Here's the drawing with two shaded views (mm, measured from the low corner). I have some questions. Round coordinates to 2 decimals unless told otherwise and drop trailing zeros. Order: outer loops, then holes, each group sorted by start corner. A loop starts at its lowest first (then second) coordinate and runs counter-clockwise, first axis right, second up. Notation, with made-up numbers: (18.5, 70) -> (47.5, 70) arc R22 ccw to (47.5, 106) -> close; hole circle Ø4 at (62.5, -6.75). An arc over 180 degrees is marked (long way). One line per question, with ' | ' between items.
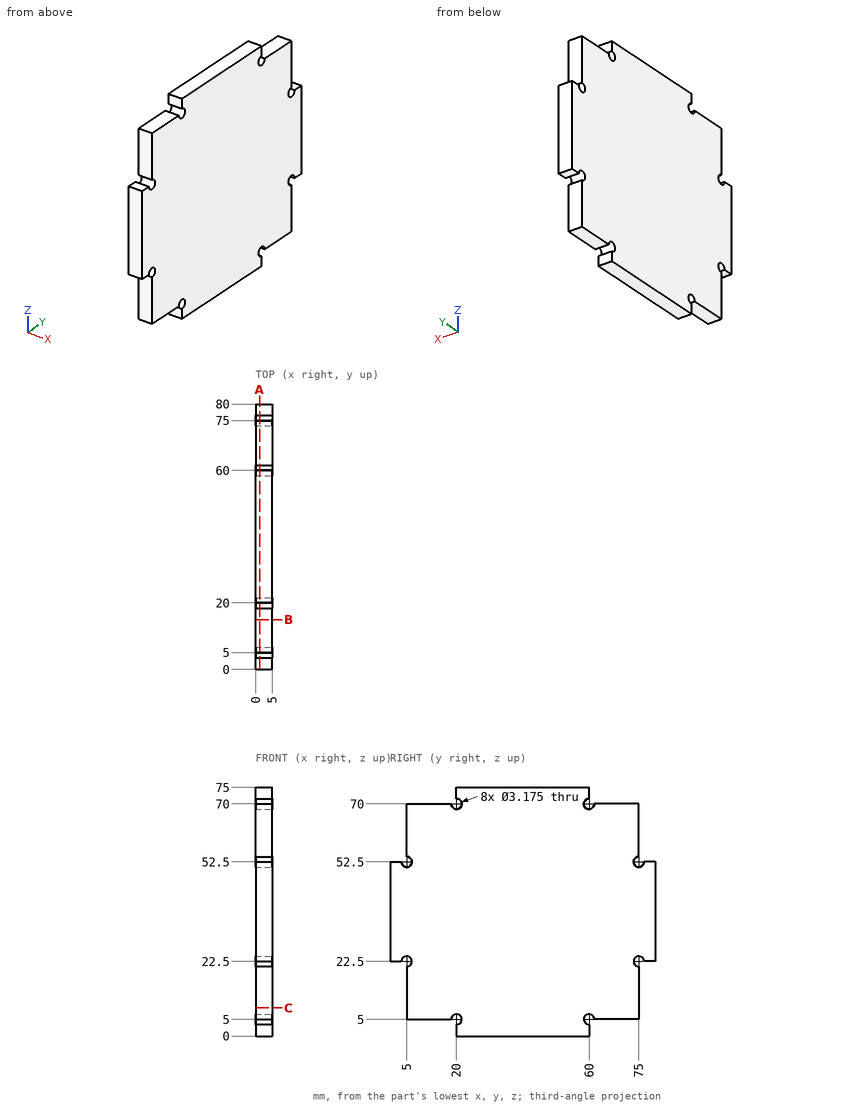
1. I need wall thicknesses on probe 1 along Z at (x, y) = (0.3, 17); probe 2 along Z at (x, y) = (4.65, 20.5); probe 3 along Y at (x, z) = (3.3, 62). Which ranges of each line are inside material? Lowest first, please.
From the geometry:
probe 1: z = 5 to 70 | probe 2: z = 0 to 3.49, 6.51 to 68.49, 71.51 to 75 | probe 3: y = 5 to 75
2. I want a section at A-A on x = 1.2. List the corners of the cut face in (y, z) for me (1 decimal).
From the geometry:
outline: (0, 22.5) -> (3.4, 22.5) arc R1.6 cw (long way) to (5, 20.9) -> (5, 5) -> (18.4, 5) arc R1.6 cw (long way) to (20, 3.4) -> (20, 0) -> (60, 0) -> (60, 3.4) arc R1.6 cw (long way) to (61.6, 5) -> (75, 5) -> (75, 20.9) arc R1.6 cw (long way) to (76.6, 22.5) -> (80, 22.5) -> (80, 52.5) -> (76.6, 52.5) arc R1.6 cw (long way) to (75, 54.1) -> (75, 70) -> (61.6, 70) arc R1.6 cw (long way) to (60, 71.6) -> (60, 75) -> (20, 75) -> (20, 71.6) arc R1.6 cw (long way) to (18.4, 70) -> (5, 70) -> (5, 54.1) arc R1.6 cw (long way) to (3.4, 52.5) -> (0, 52.5) -> close
3. I want a section at C-C on z = 8.5. List the corners of the cut face in (x, y) for me, and give its area (3 significant figures).
From the geometry:
outline: (0, 5) -> (5, 5) -> (5, 75) -> (0, 75) -> close | area: 350 mm²
4. I'm going to push flat-ended pins straight in: pin 1 (1 mm diameter, centred on x = 2, z = 73, fed in from +Y); pin 2 (2.5 mm diameter, centred on x = 3, y = 2, fed in from +Z); pin 3 (2.5 mm diameter, centred on x = 3.5, z = 10.5, fed in from -Y). Where does each tip first touch, or does it pass through?
From the geometry:
pin 1: stops at y = 60 | pin 2: stops at z = 52.5 | pin 3: stops at y = 5
5. I want a section at B-B on y = 15. List the corners of the cut face in (x, z) for me, and give its area (3 significant figures).
From the geometry:
outline: (0, 5) -> (5, 5) -> (5, 70) -> (0, 70) -> close | area: 325 mm²
